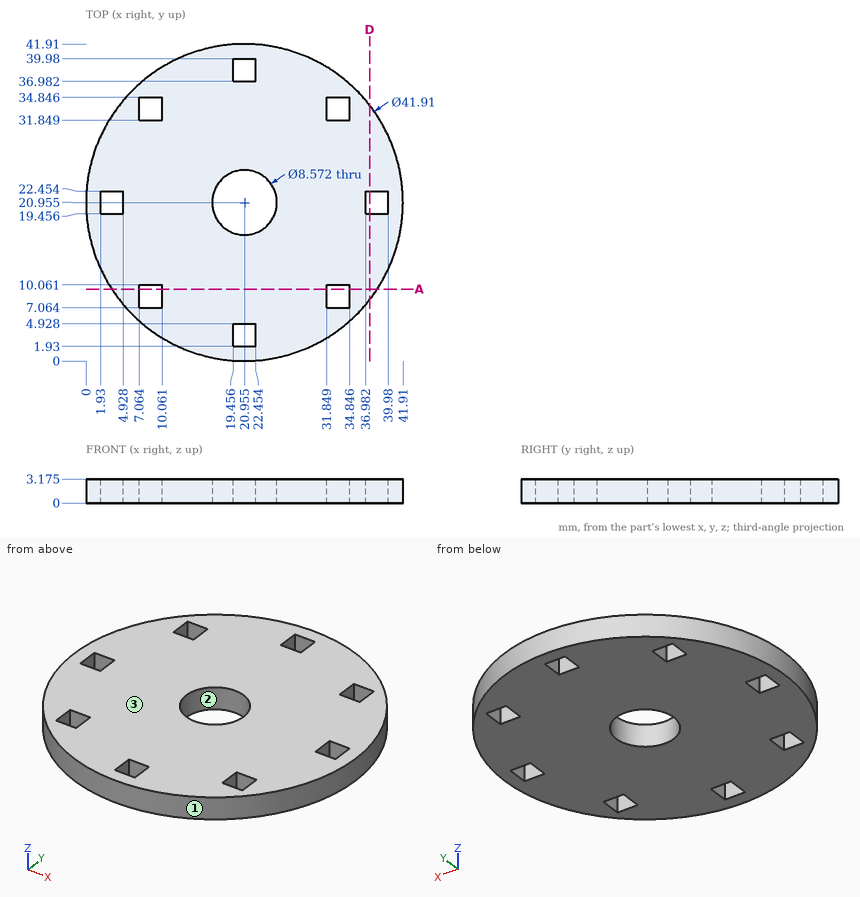
Could you check a few things on this drawing? It's one solid part, dimensions in mm from its lowest x, y, z. Coordinates: 2 decimals unless noted, no trailing zeros. Order: outer loops, then holes, each group sorted by start corner. A loop starts at its lowest first (then second) coordinate and runs counter-clockwise, first axis right, second up. Notation, with made-up numbers: M 42,25.25 L 51,25.25 A32 cw 51,63.25 Z; hole C 15.5,34.25 d1. An arc over 180 degrees is marked long. Use one line per item in the form item = value. Start each with the question number.
1. Suppose I cut it at A-A on y = 9.5. Count the separate pieces of the cut face and the enclosed holes in it.
2. Please list where these lines run through material, in increasing order: line 1 (Y direction, x = 21, z = 1.2); line 2 (X direction, y = 24.5, z = 0.45) (1 decimal); line 3 (Y direction, x = 17, z = 2.1) (1 decimal).
3. Suppose I cut it at D-D on x = 37.5. Write out the boundary of the cut face in (y, z) (1 decimal).
4. For pin 1 (1.5 mm diameter, centred on y = 35.5, z = 2, fed in from -X); pin 2 (0.9 mm diameter, centred on y = 33.5, z = 2, fed in from -X); pin 3 (4 mm diameter, centred on x = 32, y = 24, fed in from -Z); pin 4 (1.5 mm diameter, centred on x = 38.5, z = 1.5, fed in from +Y) (1 decimal), each with a flat end and sliding along its axis, tell me the tip position at first contact or that it passes through.
5. We'd pull the mould along Y, two halves only. Please class the marked faces 1, 2 and 3: +Y half, -Y half, draft (parallel to the pull), parting line (faces both ways), or undercut.
Geometry says:
q1.separate_pieces = 3
q1.enclosed_holes = 0
q2.line_1 = 0 to 1.93, 4.93 to 16.67, 25.24 to 36.98, 39.98 to 41.91
q2.line_2 = 0.3 to 18.5, 23.4 to 41.6
q2.line_3 = 0.4 to 19.3, 22.6 to 41.5
q3.outline = M 8.1,0 L 19.5,0 L 19.5,3.2 L 8.1,3.2 Z; M 22.5,0 L 33.8,0 L 33.8,3.2 L 22.5,3.2 Z
q4.pin_1 = 5.18
q4.pin_2 = 3.84
q4.pin_3 = 0
q4.pin_4 = 33.5
q5.face_1 = parting line
q5.face_2 = undercut
q5.face_3 = draft
